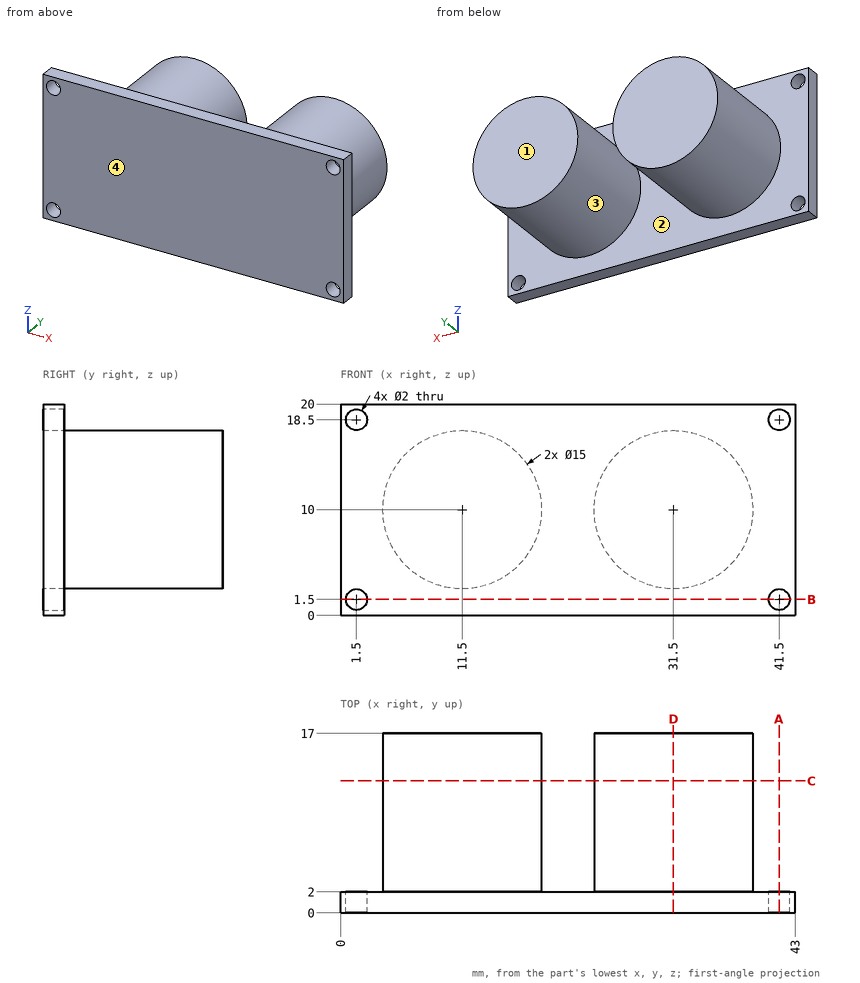
Print and shaded views of the part. All mm, measured from the part's lowest x, y and z. A direction names the side the tool comes from. Give positions to 0.01 mm unless a question says otherwise; leave off trailing zeros. Order: outer loops, then holes, each group sorted by start corner. A loop starts at its lowest first (then second) coordinate and runs counter-clockwise, first axis right, second up. Notation, with made-up numbers: (14.5, 36.5) - (59.5, 36.5) arc R24 cw to (59.5, 56.5) - close; hole circle Ø4 at (79, 37). An arc over 180 degrees is marked (long way). One line per item, written item: value.
Item 1: Slice it at D-D (x = 31.5). List the corners of the cut face in (y, z), then the cut area to 3 significant figures.
Response values:
outline: (0, 0) - (2, 0) - (2, 2.5) - (17, 2.5) - (17, 17.5) - (2, 17.5) - (2, 20) - (0, 20) - close
area: 265 mm2
Item 2: Slice it at B-B (z = 1.5). List the corners of the cut face in (x, y).
Response values:
outline: (0, 0) - (0.5, 0) - (0.5, 2) - (0, 2) - close; (2.5, 0) - (40.5, 0) - (40.5, 2) - (2.5, 2) - close; (42.5, 0) - (43, 0) - (43, 2) - (42.5, 2) - close
Item 3: Tool access for the marked faces 3 and 4: list every direction of +Z, -Z, +X, -X, +Y, -Y with a clear straight run to the whole face (end or side of a thin tool).
Response values:
face 3: +Y
face 4: +Z, -Z, +X, -X, -Y
Item 4: Pin check, flat tips, straight feed: pin 1 Ø3 at (x, z) = (1.5, 1.5) entering from +Y; pin 2 Ø1 at (x, y) = (24.5, 3.5) entering from -Z; pin 3 Ø10 at (x, y) = (25.5, 13.5) entering from +Z; pin 4 Ø2.5 at (x, z) = (41.5, 18.5) entering from -Y. Stop position of each tip, or through.
Response values:
pin 1: y = 2
pin 2: z = 6.26
pin 3: z = 17.43
pin 4: y = 0
Item 5: Wall check: line 1 (X direction, y = 1.1, z = 18.5); line 2 (X direction, y = 13, z = 9.75); line 3 (Y direction, x = 19.5, z = 3.75). Give the ranges that are in metal, low to high.
Response values:
line 1: 0 to 0.5, 2.5 to 40.5, 42.5 to 43
line 2: 4 to 19, 24 to 39
line 3: 0 to 2
Item 6: Slice it at A-A (x = 41.5). List the corners of the cut face in (y, z), then the cut area to 3 significant figures.
Response values:
outline: (0, 0) - (2, 0) - (2, 0.5) - (0, 0.5) - close; (0, 2.5) - (2, 2.5) - (2, 17.5) - (0, 17.5) - close; (0, 19.5) - (2, 19.5) - (2, 20) - (0, 20) - close
area: 32.0 mm2
Item 7: Slice it at C-C (y = 12.5). List the corners of the cut face in (x, z), then the cut area to 3 significant figures.
Response values:
outline: circle Ø15 at (11.5, 10); circle Ø15 at (31.5, 10)
area: 353 mm2
Item 8: Two-plate mould, pull along X, no slides. Class the marked faces 1 and 2: released by +X, released by -X, zero draft, split by the parting line, or undercut.
Response values:
face 1: zero draft
face 2: undercut
